Geometry: final body of the model. Coordinates: model frame, mm. A direction names the side the tool comes from. Give positions to 0.01 mm unless a question says otherwise; leave off trailing zeros. Write each loop counter-clockwise with the first axis right and the second up, starting at its lowest first coordinate (ties: lowest second). Pieces come first, ordered by that corner, then holes.
from build123d import *

# Parameters (mm, degrees)
F2_R      = 34.4044739417
F3_DEPTH  = 190.5
F6_R      = 12.7
F8_W      = 45.4750240587
F8_H      = 16.7945176363
F10_R     = 7.7759121847
F11_DEPTH = 177.8
F12_SIZE  = 5.08


# Not quite as in the source:
# - a fillet or chamfer that OpenCascade refuses, or shapes differently, is made with other operations: its cross-section is extruded or revolved along the edge and cut away or added
# - the program builds the solid bodies; features that only make, move or delete a surface that nothing else refers to are left out


with BuildPart() as f1:
    # F0 (on Right) → F1 (revolve)
    with BuildSketch(Plane.YZ):
        Polygon((38.1, -101.6), (38.1, 0), (38.1, 101.6), (0, 101.6), (0, 0), (0, -101.6), align=None)
    revolve(axis=Axis((0, 0, -50.8), (0, 0, -1)))

    # F2 (on face) → F3 (cut)
    with BuildSketch(Plane.XY.offset(101.6)):
        Circle(F2_R)
    extrude(amount=-F3_DEPTH, mode=Mode.SUBTRACT)

    # F6
    f6_edges = [f1.edges().sort_by_distance(p)[0] for p in [
        (0, -38.1, -101.6),
    ]]
    fillet(f6_edges, radius=F6_R)

    # F7: fillet of radius 5.08 on 1 edges, made by hand

    # F7_s1 → F7_t2 (revolve, cut)
    with BuildSketch(Plane.YZ):
        with BuildLine():
            ThreePointArc((38.1, 96.52), (36.6121024484, 100.1121024484), (33.02, 101.6))
            Line((33.02, 101.6), (38.1, 101.6))
            Line((38.1, 101.6), (38.1, 96.52))
        make_face()
    revolve(axis=Axis((0, 0, 101.6), (0, 0, -1)), mode=Mode.SUBTRACT)

    # F8 (on Right) → F9 (revolve)
    with BuildSketch(Plane.YZ):
        with Locations((22.7375120293, 103.7051230669)):
            Rectangle(F8_W, F8_H)
    revolve(axis=Axis((0, 0, 103.7051230669), (0, 0, -1)))

    # F10 (on face) → F11 (cut)
    with BuildSketch(Plane.XY.offset(112.1023818851)):
        with Locations((5.7727694511, 7.4173058383)):
            Circle(F10_R)
    extrude(amount=-F11_DEPTH, mode=Mode.SUBTRACT)

    # F12
    f12_edges = [f1.edges().sort_by_distance(p)[0] for p in [
        (0, -45.475024, 112.102382),
    ]]
    chamfer(f12_edges, length=F12_SIZE)


solid = f1.part
Q1. Section A-A on z = 5.5. Output: boundary loops of the cut face in (x, y).
Filled sheet:
outline: circle Ø76.2 at (0, 0); hole circle Ø68.81 at (0, 0)
Q2. Access query for faces 1 (the cylindrical face through (-23.183, -30.235, 4.493)), 2 (the flat face through (1, 1, 112.102)), 3 (the flat face through (0, 0, 95.308)). Directions: +Z, -Z, +X, -X, +Y, -Y. A direction counts if a zero-diameter tool reaches every point of the face in a straight line with its end or side. Return the directions, or none.
Filled sheet:
face 1: -Z
face 2: +Z, +X, -X, +Y, -Y
face 3: none
Q3. Pin query (flat end, axial travel): P1, Ø6, axis at x = -9.5, z = 2, coming from the +Y side; P2, Ø1.5, axis at x = -34.5, z = 11.5, coming from the +Y side; P3, Ø3, axis at x = -22.5, z = -66, coming from the +Y side. Return the tip coordinate at first contact, or that it passes through.
Filled sheet:
P1: stops at y = 37.54
P2: stops at y = 17.68
P3: stops at y = 31.79
Q4. Ray query, line 1 along Z through (x, y) = (-17, 14); line 2 along Y through (x, z) = (0, -8); line 3 along Z through (x, y) = (31, 5.5). Return the intervals inside material, ascending.
Filled sheet:
line 1: z = -101.6 to -88.9, 95.31 to 112.1
line 2: y = -38.1 to -34.4, 34.4 to 38.1
line 3: z = -100.05 to -88.9, 95.31 to 112.1
Q5. Pull-direction query (Z, two-part tool) for faces 4 (the flat face through (-37, 10, 95.308)), 5 (the cylindrical face through (4.087, -0.174, 103.823)), 6 (the flat face through (0, 0, -88.9)), 7 (the conical face through (-24.73, -32.252, 111.856)); classes: released by +Z, released by -Z, zero draft, split by the parting line, or undercut.
Filled sheet:
face 4: released by -Z
face 5: zero draft
face 6: undercut
face 7: released by +Z
Q6. Section B-B on x = 0. Output: boundary loops of the cut face in (y, z), plus the area to 3 significant figures.
Filled sheet:
outline: (-45.48, 95.31) - (-38.1, 95.31) - (-38.1, -88.9) arc R12.7 ccw to (-25.4, -101.6) - (25.4, -101.6) arc R12.7 ccw to (38.1, -88.9) - (38.1, 95.31) - (45.48, 95.31) - (45.48, 107.02) - (40.4, 112.1) - (12.63, 112.1) - (12.63, 95.31) - (34.4, 95.31) - (34.4, -88.9) - (-34.4, -88.9) - (-34.4, 95.31) - (2.21, 95.31) - (2.21, 112.1) - (-40.4, 112.1) - (-45.48, 107.02) - close
area: 3,590 mm2
